from build123d import *

# Parameters (mm, degrees)
SKETCH1_R           = 3.45
SKETCH1_R_2         = 6.5
BOSS_EXTRUDE1_DEPTH = 6
BOSS_EXTRUDE2_DEPTH = 6
BOSS_EXTRUDE4_DEPTH = 6


with BuildPart() as part:
    # Sketch1 → Boss-Extrude1 (new body)
    with BuildSketch(Plane(origin=(0, 0, 0), x_dir=(1, 0, 0), z_dir=(0, 1, 0))):
        with BuildLine():
            Line((-4.45, 0), (0, 60))
            Line((0, 60), (4.45, 0))
            Line((4.45, 0), (7.332848837, -13.425411822))
            ThreePointArc((7.332848837, -13.425411822), (0, -22.5), (-7.332848837, -13.425411822))
            Line((-7.332848837, -13.425411822), (-4.45, 0))
        make_face()
        with Locations(Location((0, 0, 0), (0, 0, 270))):
            Circle(SKETCH1_R, mode=Mode.SUBTRACT)
        with Locations(Location((0, -15, 0), (0, 0, 270))):
            Circle(SKETCH1_R_2, mode=Mode.SUBTRACT)
        with BuildLine():
            Line((-5.56959306, -9.977089176), (-3.890910153, -2.159471736))
            ThreePointArc((-3.890910153, -2.159471736), (0, -4.45), (3.890910153, -2.159471736))
            Line((3.890910153, -2.159471736), (5.56959306, -9.977089176))
            ThreePointArc((5.56959306, -9.977089176), (0, -7.5), (-5.56959306, -9.977089176))
        make_face(mode=Mode.SUBTRACT)
        with BuildLine():
            Line((-3.219404352, 3.072122332), (0, 46.479821455))
            Line((0, 46.479821455), (3.219404352, 3.072122332))
            ThreePointArc((3.219404352, 3.072122332), (0, 4.45), (-3.219404352, 3.072122332))
        make_face(mode=Mode.SUBTRACT)
    extrude(amount=BOSS_EXTRUDE1_DEPTH)

    # Sketch3 → Boss-Extrude2 (add)
    with BuildSketch(Plane(origin=(0, 0, 0), x_dir=(1, 0, 0), z_dir=(0, 1, 0))):
        with BuildLine():
            Line((-2.424610287, 13.788446793), (-2.501099218, 12.757135364))
            ThreePointArc((-2.501099218, 12.757135364), (0, 13), (2.501099218, 12.757135364))
            Line((2.501099218, 12.757135364), (2.424610287, 13.788446793))
            ThreePointArc((2.424610287, 13.788446793), (0, 14), (-2.424610287, 13.788446793))
        make_face()
        with BuildLine():
            Line((-1.971141851, 19.902627962), (-2.046283127, 18.889487165))
            ThreePointArc((-2.046283127, 18.889487165), (0, 19), (2.046283127, 18.889487165))
            Line((2.046283127, 18.889487165), (1.971141851, 19.902627962))
            ThreePointArc((1.971141851, 19.902627962), (0, 20), (-1.971141851, 19.902627962))
        make_face()
        with BuildLine():
            Line((-1.518937845, 25.999760627), (-1.593540779, 24.993878368))
            ThreePointArc((-1.593540779, 24.993878368), (0, 25.044626731), (1.593540779, 24.993878368))
            Line((1.593540779, 24.993878368), (1.518937845, 25.999760627))
            ThreePointArc((1.518937845, 25.999760627), (0, 26.044091937), (-1.518937845, 25.999760627))
        make_face()
        with BuildLine():
            Line((-1.072221947, 32.022896321), (-1.146588325, 31.020203596))
            ThreePointArc((-1.146588325, 31.020203596), (0, 31.041386823), (1.146588325, 31.020203596))
            Line((1.146588325, 31.020203596), (1.072221947, 32.022896321))
            ThreePointArc((1.072221947, 32.022896321), (0, 32.040841885), (-1.072221947, 32.022896321))
        make_face()
        with BuildLine():
            Line((-0.626517111, 38.032399738), (-0.700752129, 37.031478145))
            ThreePointArc((-0.700752129, 37.031478145), (0, 37.038107769), (0.700752129, 37.031478145))
            Line((0.700752129, 37.031478145), (0.626517111, 38.032399738))
            ThreePointArc((0.626517111, 38.032399738), (0, 38.037559774), (-0.626517111, 38.032399738))
        make_face()
        with BuildLine():
            Line((-0.181406226, 44.033894812), (-0.255560758, 43.034058423))
            ThreePointArc((-0.255560758, 43.034058423), (0, 43.034817249), (0.255560758, 43.034058423))
            Line((0.255560758, 43.034058423), (0.181406226, 44.033894812))
            ThreePointArc((0.181406226, 44.033894812), (0, 44.034268479), (-0.181406226, 44.033894812))
        make_face()
        with BuildLine():
            ThreePointArc((4.761236709, -19.425), (5.270605983, -18.804038982), (5.699506558, -18.125))
            ThreePointArc((5.699506558, -18.125), (0, -19), (-5.699506558, -18.125))
            ThreePointArc((-5.699506558, -18.125), (-5.270605983, -18.804038982), (-4.761236709, -19.425))
            ThreePointArc((-4.761236709, -19.425), (0, -20), (4.761236709, -19.425))
        make_face()
        with BuildLine():
            ThreePointArc((-5.614657158, -11.725), (-5.849946188, -12.166604581), (-6.050568155, -12.625))
            ThreePointArc((-6.050568155, -12.625), (0, -14), (6.050568155, -12.625))
            ThreePointArc((6.050568155, -12.625), (5.849946188, -12.166604581), (5.614657158, -11.725))
            ThreePointArc((5.614657158, -11.725), (0, -13), (-5.614657158, -11.725))
        make_face()
    extrude(amount=BOSS_EXTRUDE2_DEPTH)

    # Sketch5 → Boss-Extrude4 (add)
    with BuildSketch(Plane(origin=(0, 0, 0), x_dir=(1, 0, 0), z_dir=(0, 1, 0))):
        with BuildLine():
            Line((9.212671688, 27.282460114), (11, 25))
            ThreePointArc((11, 25), (10.891360502, 26.004918608), (10.570462139, 26.963400841))
            ThreePointArc((10.570462139, 26.963400841), (9.696667899, 28.24931958), (8.451309377, 29.180010468))
            ThreePointArc((8.451309377, 29.180010468), (7.63085583, 29.509197363), (6.763286857, 29.67899757))
            ThreePointArc((6.763286857, 29.67899757), (6.1879429, 29.700797107), (5.614247813, 29.652116139))
            ThreePointArc((5.614247813, 29.652116139), (4.779917704, 29.450310868), (3.996176977, 29.100192931))
            ThreePointArc((3.996176977, 29.100192931), (3.558596441, 28.82174206), (3.154345742, 28.496791317))
            ThreePointArc((3.154345742, 28.496791317), (2.463689343, 27.721817132), (1.959907971, 26.814185279))
            Line((1.959907971, 26.814185279), (2.094460046, 25))
            Line((2.094460046, 25), (2.595833333, 25))
            ThreePointArc((2.595833333, 25), (5.090697751, 28.499720488), (9.212671688, 27.282460114))
        make_face()
        with BuildLine():
            Line((1.647961612, 31.020203596), (1.749949079, 29.645091687))
            Line((1.749949079, 29.645091687), (3.154345742, 28.496791317))
            ThreePointArc((3.154345742, 28.496791317), (3.558596441, 28.82174206), (3.996176977, 29.100192931))
            Line((3.996176977, 29.100192931), (1.647961612, 31.020203596))
        make_face()
        with BuildLine():
            ThreePointArc((5.614247813, 29.652116139), (6.1879429, 29.700797107), (6.763286857, 29.67899757))
            Line((6.763286857, 29.67899757), (1.037132306, 39.256104353))
            Line((1.037132306, 39.256104353), (1.202125417, 37.031478145))
            Line((1.202125417, 37.031478145), (5.614247813, 29.652116139))
        make_face()
        with BuildLine():
            ThreePointArc((8.451309377, 29.180010468), (9.696667899, 28.24931958), (10.570462139, 26.963400841))
            Line((10.570462139, 26.963400841), (0.289570354, 49.335591342))
            Line((0.289570354, 49.335591342), (0.501373288, 46.479821455))
            Line((0.501373288, 46.479821455), (8.451309377, 29.180010468))
        make_face()
        with BuildLine():
            Line((1.749949079, 29.645091687), (1.959907971, 26.814185279))
            ThreePointArc((1.959907971, 26.814185279), (2.463689343, 27.721817132), (3.154345742, 28.496791317))
            Line((3.154345742, 28.496791317), (1.749949079, 29.645091687))
        make_face()
    boss_extrude4 = extrude(amount=BOSS_EXTRUDE4_DEPTH)

    # Mirror1: Boss-Extrude4 across plane
    add(boss_extrude4.mirror(Plane(origin=(0, 0, 0), x_dir=(0, 0, 1), z_dir=(1, 0, 0))))


solid = part.part
Here's how the part is built. I have some questions about the finished solid (model axes, mm). A direction names the side the tool comes from. Give positions to 0.01 mm unless a question says otherwise; leave off trailing zeros. Order: outer loops, then holes, each group sorted by start corner. A loop starts at its lowest first (then second) coordinate and runs counter-clockwise, first axis right, second up. Notation, with made-up numbers: (-40, 42) -> (-27, 42) arc R14 cw to (-27, 69) -> close; hole circle Ø7 at (-35.5, 0.25). An arc over 180 degrees is marked (long way). Use a Markdown table: item, result. Add a question column.
Item 1: I need wall thicknesses on line 1 (X direction, y = 4.85, z = 0); line 2 (X direction, y = 2.6, z = 5.5); line 3 (Z direction, x = 8, y = 4.7). Which ranges of each line are inside material? Lowest first, please.
Item 2: Imagine slicing it at B-B on z = -6.5. Please give me the cut outline in (x, y).
Item 3: If we mould it in two halves opening along X, with no side actions, what happens to faces 1 (the face through (5.87, 2.96, 6.62)), 2 (the face through (-4.724, 2.958, -37.291)), 3 (the face through (-5.912, 2.958, 6.807))? For each: pulls with the +X half, pulls with the -X half, needs draft (parallel to the pull), parting line crosses it, or undercut.
Item 4: Imagine slicing it at A-A on z = 15. Please give me the cut outline in (x, y).
Item 5: Imagine slicing it at D-D on z = -54. Please give me the cut outline in (x, y) (3 decimals).
Item 6: For faces 4 (the face through (3.51, 2.96, -12.68)), 5 (the face through (-0.022, 2.958, -25.045)), 6 (the face through (-10.09, 2.96, -26.16)), which set-ups out of +Z, -Z, +X, -X, +Y, -Y let a thin tool reach every point of the face, with its end or its side?
Item 7: Will these pins go through, and if not, where does the flat tip stop? pin 1 (3 mm diameter, centred on x = -7, z = -42, fed in from -Y); pin 2 (1.5 mm diameter, centred on x = -7.5, y = 2, fed in from -Z); pin 3 (3 mm diameter, centred on y = 2.5, z = -28, fed in from -X).
Item 8: Imagine slicing it at C-C on y = 3.35. Give the number of separate pieces and of enclosed holes in the cut face, plus the area to 3 significant figures.
Data:
| question | item | result |
|---|---|---|
| 1 | line 1 | x = -4.45 to -3.45, 3.45 to 4.45 |
| 1 | line 2 | x = -5.63 to -4.61, 4.61 to 5.63 |
| 1 | line 3 | z = -32.56 to -30.16, -29.38 to -28.29 |
| 2 | outline | (-3.97, 0) -> (-2.97, 0) -> (-2.97, 6) -> (-3.97, 6) -> close; (2.97, 0) -> (3.97, 0) -> (3.97, 6) -> (2.97, 6) -> close |
| 3 | face 1 | pulls with the +X half |
| 3 | face 2 | undercut |
| 3 | face 3 | pulls with the -X half |
| 4 | outline | (-7.5, 0) -> (-6.5, 0) -> (-6.5, 6) -> (-7.5, 6) -> close; (6.5, 0) -> (7.5, 0) -> (7.5, 6) -> (6.5, 6) -> close |
| 5 | outline | (-0.445, 0) -> (0.445, 0) -> (0.445, 6) -> (-0.445, 6) -> close |
| 6 | face 4 | +X, +Y, -Y |
| 6 | face 5 | +Y, -Y |
| 6 | face 6 | +Z, +Y, -Y |
| 7 | pin 1 | passes through |
| 7 | pin 2 | stops at z = -35.28 |
| 7 | pin 3 | stops at x = -10.75 |
| 8 | separate pieces | 1 |
| 8 | enclosed holes | 16 |
| 8 | area | 313 mm² |
